For this review, take the finished solid that the model builds, in its own axes (mm). Face numbers are marked on the shaded views. A direction names the side the tool comes from. Round coordinates to 2 decimals unless told otherwise and drop trailing zeros. Write each loop counter-clockwise with the first axis right and the second up, starting at its lowest first coordinate (ties: lowest second). Pieces come first, ordered by that corner, then holes. Notation, with made-up numbers: (34, 49) -> (70, 49) arc R19 ccw to (70, 79) -> close; hole circle Ø7 at (75.25, -17). An arc over 180 degrees is marked (long way). Answer in a Markdown table with one row per item.
from build123d import *

# Parameters (mm, degrees)
F0_R         = 12.875
F1_DEPTH     = 5.8
F2_R         = 9.875
F3_DEPTH     = 12
F5_DEPTH     = 5
F7_W         = 30
F7_H         = 30
F7_W_2       = 18
F7_H_2       = 27
F8_DEPTH     = 10
F15_W        = 17
F15_H        = 30
F16_DEPTH    = 15
F18_R        = 1.5
F19_T1_DEPTH = 5.8


# Not quite as in the source:
# - a fillet or chamfer that OpenCascade refuses, or shapes differently, is made with other operations: its cross-section is extruded or revolved along the edge and cut away or added
# - a feature names something its author has since deleted; it is built from what else it names


with BuildPart() as f1:
    # F0 (on Top) → F1 (new body)
    with BuildSketch(Plane.XY):
        Circle(F0_R)
    extrude(amount=-F1_DEPTH)

    # F2 (on Top) → F3 (join)
    with BuildSketch(Plane.XY):
        Circle(F2_R)
    extrude(amount=F3_DEPTH)


with BuildPart() as f5:
    # F4 (on Top) → F5 (new body)
    with BuildSketch(Plane.XY):
        with BuildLine():
            ThreePointArc((-2.19192449, 8.7487287819), (-0.0332522533, 9.0190732649), (2.1273547272, 8.7646534521))
            ThreePointArc((2.1273547272, 8.7646534521), (-0.0376344683, 10.2076699565), (-2.19192449, 8.7487287819))
        make_face()
    extrude(amount=F5_DEPTH)


with BuildPart() as f6_1:
    # F6: instance of F5
    add(f5.part.mirror(Plane.XZ))


with BuildPart() as f8:
    # F7 (on Top) → F8 (new body, symmetric)
    with BuildSketch(Plane.XY):
        Rectangle(F7_W, F7_H)
        Rectangle(F7_W_2, F7_H_2, mode=Mode.SUBTRACT)
    extrude(amount=F8_DEPTH, both=True)


with BuildPart() as f1_1:
    add(f1.part)

    # F9: cut F8
    add(f8.part, mode=Mode.SUBTRACT)


with BuildPart() as f16:
    # F15 (on face) → F16 (new body)
    with BuildSketch(Plane(origin=(0, 0, -10.8), x_dir=(1, 0, 0), z_dir=(0, 0, -1))):
        Rectangle(F15_W, F15_H)
    extrude(amount=-F16_DEPTH)

    # F17: cut F6_1, F5, F1
    add(f6_1.part, mode=Mode.SUBTRACT)
    add(f5.part, mode=Mode.SUBTRACT)
    add(f1_1.part, mode=Mode.SUBTRACT)

    # F18
    f18_edges = [f16.edges().sort_by_distance(p)[0] for p in [
        (8.5, -5.026492, 2.1),
        (8.5, 5.026492, 2.1),
        (-8.5, 5.026492, 2.1),
        (-8.5, -5.026492, 2.1),
    ]]
    fillet(f18_edges, radius=F18_R)

    # F19: fillet of radius 0.5 on 4 edges, made by hand

    # F19_s2 → F19_t1 (cut)
    with BuildSketch(Plane.XY.offset(-5.8)):
        with BuildLine():
            add(Edge.make_bspline(
                [(-7.7009345794, 10.3180052143), (-8.5, 9.7216156603), (-8.5, 10.718704446)],
                knots=[0, 0, 0, 1, 1, 1], degree=2, weights=[1, 1, 1]))
            Line((-8.5, 10.718704446), (-8.5, 9.6703477187))
            ThreePointArc((-8.5, 9.6703477187), (-8.106937484, 10.0021592484), (-7.7009345794, 10.3180052143))
        make_face()
        with BuildLine():
            add(Edge.make_bspline(
                [(-7.7009345794, -10.3180052143), (-8.5, -9.7216156603), (-8.5, -10.718704446)],
                knots=[0, 0, 0, 1, 1, 1], degree=2, weights=[1, 1, 1]))
            Line((-8.5, -10.718704446), (-8.5, -9.6703477187))
            ThreePointArc((-8.5, -9.6703477187), (-8.106937484, -10.0021592484), (-7.7009345794, -10.3180052143))
        make_face()
        with BuildLine():
            add(Edge.make_bspline(
                [(8.5, 10.718704446), (8.5, 9.7216156603), (7.7009345794, 10.3180052143)],
                knots=[0, 0, 0, 1, 1, 1], degree=2, weights=[1, 1, 1]))
            ThreePointArc((7.7009345794, 10.3180052143), (8.106937484, 10.0021592484), (8.5, 9.6703477187))
            Line((8.5, 9.6703477187), (8.5, 10.718704446))
        make_face()
        with BuildLine():
            add(Edge.make_bspline(
                [(8.5, -10.718704446), (8.5, -9.7216156603), (7.7009345794, -10.3180052143)],
                knots=[0, 0, 0, 1, 1, 1], degree=2, weights=[1, 1, 1]))
            ThreePointArc((7.7009345794, -10.3180052143), (8.106937484, -10.0021592484), (8.5, -9.6703477187))
            Line((8.5, -9.6703477187), (8.5, -10.718704446))
        make_face()
    extrude(amount=F19_T1_DEPTH, mode=Mode.SUBTRACT)


solid = f16.part
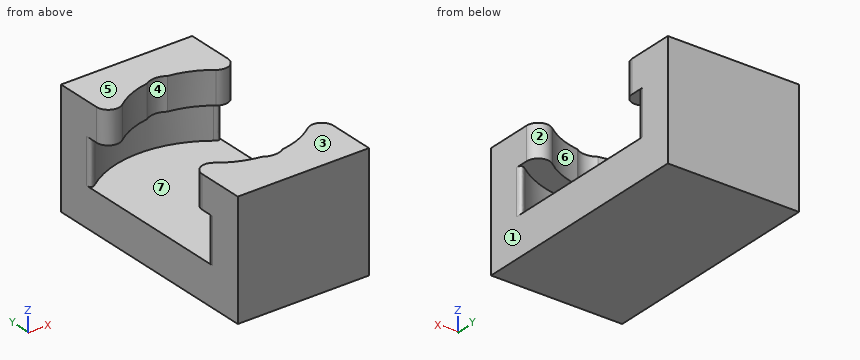
1) Mouldability with a two-part tool opening along X and no side actions: class the marked faces 1, 2, 3 and 4 as pulls with the +X half, pulls with the -X half, needs draft (parallel to the pull), parting line crosses it, or undercut.
Solved:
| item | result |
|---|---|
| face 1 | pulls with the +X half |
| face 2 | undercut |
| face 3 | needs draft |
| face 4 | undercut |
2) Consider section C-C on x = -3.25. State the section outline as (y, z) points, then the cut area to 3 significant figures.
Solved:
| item | result |
|---|---|
| outline | (-15, -10.8) -> (15, -10.8) -> (15, 4.2) -> (9.32, 4.2) -> (9.32, 0) -> (12.46, 0) -> (12.46, -5.8) -> (-12.46, -5.8) -> (-12.46, 0) -> (-9.32, 0) -> (-9.32, 4.2) -> (-15, 4.2) -> close |
| area | 227 mm² |
3) Consider section D-D on y = 3. State the section outline as (x, z) points, then the cut area to 3 significant figures.
Solved:
| item | result |
|---|---|
| outline | (-8.5, -10.8) -> (8.5, -10.8) -> (8.5, -5.8) -> (-8.5, -5.8) -> close |
| area | 85.0 mm² |
4) Clearance check with a flat-ended pin moving along its axis: pin 1 Ø5 at (x, y) = (-3, 4.5) entering from +Z. State where the tip first meets the part, or that it passes through.
Solved:
| item | result |
|---|---|
| pin 1 | z = -5.8 |
5) Consider section A-A on z = 1.25. State the section outline as (x, y) points (3 decimals), then the cut area to 3 significant figures.
Solved:
| item | result |
|---|---|
| outline | (-8.5, -15) -> (8.5, -15) -> (8.5, -8.966) arc R1.5 ccw to (6.077, -7.784) arc R9.875 cw to (1.305, -9.788) arc R2.333 cw to (-1.377, -9.778) arc R9.875 cw to (-6.077, -7.784) arc R1.5 ccw to (-8.5, -8.966) -> close; (-8.5, 8.966) arc R1.5 ccw to (-6.077, 7.784) arc R9.875 cw to (-1.377, 9.778) arc R2.333 cw to (1.305, 9.788) arc R9.875 cw to (6.077, 7.784) arc R1.5 ccw to (8.5, 8.966) -> (8.5, 15) -> (-8.5, 15) -> close |
| area | 210 mm² |
6) For line 1 (Z direction, x = -2.5, y = -10); line 2 (Z direction, x = 3.5, y = -8.25); line 3 (Y direction, x = 6.75, z = -0.25), list the stretches that pass through material, from the lowest coordinate up. Write a range as [from, to].
Solved:
| item | result |
|---|---|
| line 1 | [-10.8, -5.8], [0, 4.2] |
| line 2 | [-10.8, -5.8] |
| line 3 | [-15, -10.96], [10.96, 15] |
7) Consider section B-B on y = -11.5. State the section outline as (x, z) points, then the cut area to 3 significant figures.
Solved:
| item | result |
|---|---|
| outline | (-8.5, -10.8) -> (8.5, -10.8) -> (8.5, 4.2) -> (-8.5, 4.2) -> close; hole (-5.79, -5.8) -> (5.79, -5.8) -> (5.79, 0) -> (-5.79, 0) -> close |
| area | 188 mm² |
8) For the marked faces 5, 6 and 7, list the 3-axis set-ups (+Z, -Z, +X, -X, +Y, -Y) from which the entire face can be reached by the end or side of a thin tool; tool diameter is ignored.
Solved:
| item | result |
|---|---|
| face 5 | +Z, +X, -X, +Y, -Y |
| face 6 | +Z |
| face 7 | none |
